Build history of the part. All positions in model axes, mm. Face numbers are marked on the shaded views. A direction names the side the tool comes from. Round coordinates to 2 decimals unless told otherwise and drop trailing zeros. Write each loop counter-clockwise with the first axis right and the second up, starting at its lowest first coordinate (ties: lowest second). Pieces come first, ordered by that corner, then holes. Notation, with made-up numbers: M 57,83 L 81,83 A29 ccw 81,119 Z; hole C 2,-27 d9. An arc over 180 degrees is marked long. Write item = value, one per line. Start each with the question number.
Q1. Band-saw the part on C-C on z = 0.7. Write the cut outline in (x, y).
Q2. Probe L1, parallel to Y at x = 3.5, z = 4; L2, parallel to Z at x = 1.25, y = 91.75; L3, parallel to X at y = 88.5, z = 1.1. List the from-to ranges inside material, lowest first.
Q3. Band-saw the part on B-B on x = -2.5. Write the cut outline in (y, z).
Q4. Drop flat-ended pins along their axis: P1, Ø1.5, axis at y = 92, z = 1, coming from the -X side; P2, Ø1.2, axis at x = -1.5, z = 2, coming from the +Y side; P3, Ø3.5, axis at x = 0.5, y = 84, coming from the +Z side. Give the stop position or say it passes through.
Q5. Band-saw the part on D-D on y = 83.5. Write the cut outline in (x, z), plus the area to 3 significant figures.
Q6. Tool access for the marked faces 1, 2 and 3: list every direction of +Z, -Z, +X, -X, +Y, -Y with a clear straight run to the whole face (end or side of a thin tool).
Q7. Band-saw the part on A-A on y = 98.25. Write the cut outline in (x, z), plus the area to 3 significant figures.
```python
from build123d import *

# Parameters (mm, degrees)
EXTRUDE1_DEPTH     = 4.9
EXTRUDE2_DEPTH     = 0.9
SKETCH3_R          = 1.3462
CUT_EXTRUDE2_DEPTH = 5.9


with BuildPart() as part:
    # Sketch1 → Extrude1 (new body)
    with BuildSketch(Plane.XY):
        Polygon((-6.583958388, 90.87662316), (6.583958388, 90.87662316), (5.632133126, 85.929746212), (-5.632133126, 85.929746212), align=None)
    extrude(amount=EXTRUDE1_DEPTH)

    # Sketch2 → Extrude2 (add)
    with BuildSketch(Plane(origin=(0, 0, 0), x_dir=(-1, 0, 0), z_dir=(0, 0, -1))):
        with BuildLine():
            Line((8.178395959, 99.163319022), (6.538639227, 90.641088001))
            ThreePointArc((6.538639227, 90.641088001), (0, 90.87662316), (-6.538639227, 90.641088001))
            Line((-6.538639227, 90.641088001), (-8.178395959, 99.163319022))
            ThreePointArc((-8.178395959, 99.163319022), (0, 99.5), (8.178395959, 99.163319022))
        make_face()
        with BuildLine():
            Line((5.632133126, 85.929746212), (4.760567707, 81.4))
            Line((4.760567707, 81.4), (-4.760567707, 81.4))
            Line((-4.760567707, 81.4), (-5.632133126, 85.929746212))
            ThreePointArc((-5.632133126, 85.929746212), (0, 86.11412316), (5.632133126, 85.929746212))
        make_face()
    extrude(amount=-EXTRUDE2_DEPTH)

    # Sketch3 → Cut-Extrude2 (cut, through all)
    with BuildSketch(Plane.XY):
        with Locations(Location((-1.705972729, 97.735112202, 0), (0, 0, 180))):  # turned: the seam where the file's is
            Circle(SKETCH3_R)
        with BuildLine():
            Line((-1.069188916, 83.994208969), (-1.051733851, 82.994208969))
            ThreePointArc((-1.051733851, 82.994208969), (-1.441621981, 82.590467992), (-1.845362959, 82.980356122))
            Line((-1.845362959, 82.980356122), (-1.862818024, 83.980356122))
            ThreePointArc((-1.862818024, 83.980356122), (-1.472929894, 84.3840971), (-1.069188916, 83.994208969))
        make_face()
    extrude(amount=CUT_EXTRUDE2_DEPTH, mode=Mode.SUBTRACT)


solid = part.part
```
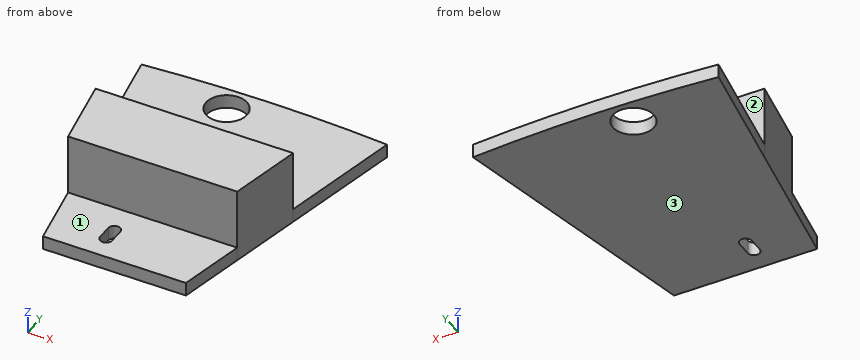
Conclusion:
q1.outline = M -8.18,99.16 L -4.76,81.4 L 4.76,81.4 L 8.18,99.16 A99.5 ccw Z; hole C -1.71,97.74 d2.69; hole M -1.86,83.98 L -1.85,82.98 A0.4 ccw -1.05,82.99 L -1.07,83.99 A0.4 ccw Z
q2.L1 = 85.93 to 90.88
q2.L2 = 0 to 0.9
q2.L3 = -6.13 to 6.13
q3.outline = M 81.4,0 L 96.65,0 L 96.65,0.9 L 90.88,0.9 L 90.88,4.9 L 85.93,4.9 L 85.93,0.9 L 81.4,0.9 Z; M 98.82,0 L 99.47,0 L 99.47,0.9 L 98.82,0.9 Z
q4.P1 = -6.94
q4.P2 = 90.88
q4.P3 = 0.9
q5.outline = M -5.16,0 L -1.85,0 L -1.85,0.9 L -5.16,0.9 Z; M -1.06,0 L 5.16,0 L 5.16,0.9 L -1.06,0.9 Z
q5.area = 8.58 mm^2
q6.face_1 = +Z, +X, -X, -Y
q6.face_2 = +Z, +X, -X, +Y
q6.face_3 = -Z, +X, -X, +Y, -Y
q7.outline = M -8,0 L -2.95,0 L -2.95,0.9 L -8,0.9 Z; M -0.46,0 L 8,0 L 8,0.9 L -0.46,0.9 Z
q7.area = 12.2 mm^2
